from build123d import *

# Parameters (mm, degrees)
BOSS_EXTRUDE1_DEPTH = 5.08
CUT_EXTRUDE1_DEPTH  = 2.413
SKETCH8_R           = 1.524
CUT_EXTRUDE2_DEPTH  = 2.667


with BuildPart() as part:
    # Sketch1 → Boss-Extrude1 (new body)
    with BuildSketch(Plane(origin=(0, 0, 0), x_dir=(1, 0, 0), z_dir=(0, 1, 0))):
        Polygon((41.520544409, 0), (-41.520544409, 0), (-41.520544409, -3.81), (-39.615544409, -3.81), (-39.615544409, -7.112), (-44.695544409, -7.112), (-44.695544409, -3.81), (-42.790544409, -3.81), (-42.790544409, 0), (-56.515, 0), (-56.515, 107.95), (-51.435, 107.95), (-51.435, 5.08), (51.435, 5.08), (51.435, 107.95), (56.515, 107.95), (56.515, 0), (42.790544409, 0), (42.790544409, -4.019776581), (47.235544409, -4.019776581), (47.235544409, -11.639776581), (37.075544409, -11.639776581), (37.075544409, -4.019776581), (41.520544409, -4.019776581), align=None)
    extrude(amount=BOSS_EXTRUDE1_DEPTH)

    # Sketch2 → Cut-Extrude1 (cut)
    with BuildSketch(Plane(origin=(0, 5.08, 0), x_dir=(1, 0, 0), z_dir=(0, 1, 0))):
        Polygon((40.322457304, -4.654776581), (38.4893702, -7.829776581), (40.322457304, -11.004776581), (43.988631514, -11.004776581), (45.821718619, -7.829776581), (43.988631514, -4.654776581), align=None)
    extrude(amount=-CUT_EXTRUDE1_DEPTH, mode=Mode.SUBTRACT)

    # Sketch8 → Cut-Extrude2 (cut)
    with BuildSketch(Plane(origin=(0, 2.667, 0), x_dir=(1, 0, 0), z_dir=(0, 1, 0))):
        with Locations(Location((42.155544409, -7.829776581, 0), (0, 0, 270))):
            Circle(SKETCH8_R)
    extrude(amount=-CUT_EXTRUDE2_DEPTH, mode=Mode.SUBTRACT)


solid = part.part
Read the model definition and answer for the solid it produces. Units are mm, in the model's axes. A direction names the side the tool comes from. Coordinates: 2 decimals unless noted, no trailing zeros. Loops run counter-clockwise (first coordinate to the right, second up) from the corner with the lowest first, then second, coordinate; pieces in that order, holes last. Notation, with made-up numbers: (-35, 87) -> (-14, 87) arc R25 ccw to (-14, 110) -> close; hole circle Ø4 at (12, -32). An arc over 180 degrees is marked (long way). Write item = value, one per line. Start each with the question number.
1) For faces 1 (the face through (44, 2.667, 8)), 2 (the face through (41.521, 3, 2)), 3 (the face through (37.076, 3, 8)), 4 (the face through (50, 3, 0)), determine the directions among +Z, -Z, +X, -X, +Y, -Y from which every point of the face is accessible in a straight line to the end or side of a thin tool.
2) Find the intervals of material crossed by L1, parallel to X at y = 4.2, z = -13 (3 decimals); L2, parallel to Z at x = -49.5, y = 4.75; L3, parallel to X at y = 2.15, z = 1, in increasing order. Write a range as from..to.
3) Given P1, Ø1, axis at x = -43.5, y = 3, coming from the -Z side; P2, Ø1, axis at y = 3, z = 5, coming from the +X side; P3, Ø7, axis at x = 41.5, z = 7.5, coming from the +Y side; P4, Ø2.5, axis at x = -43, y = 1.5, coming from the +Z side, each flat-ended and moving along its own axis, determine where each tip first touches the part or whether it passes through.
4) The part is cut by section A-A, the plane z = -96. Determine the outline of the cut face in (x, y) (3 decimals).
5) The part is cut by section C-C, the plane x = 1. Determine the outline of the cut face in (y, z), plus the area to 3 significant figures.
6) The mould has two halves that part along X. Classify faces 5 (the face through (39, 3, 4.02)), 6 (the face through (-42, 3, 7.112)), 7 (the face through (47.236, 3, 8)), 8 (the face through (-1, 3, -5.08)): pulls with the +X half, pulls with the -X half, needs draft (parallel to the pull), parting line crosses it, or undercut.
Result:
q1.face_1 = +Y
q1.face_2 = +Y, -Y
q1.face_3 = +Z, +Y, -Y
q1.face_4 = +X, +Y, -Y
q2.L1 = -56.515..-51.435, 51.435..56.515
q2.L2 = -5.08..0
q2.L3 = -42.79..-41.52, 41.52..42.79
q3.P1 = -5.08
q3.P2 = 47.24
q3.P3 = 5.08
q3.P4 = 7.11
q4.outline = (-56.515, 0) -> (-51.435, 0) -> (-51.435, 5.08) -> (-56.515, 5.08) -> close; (51.435, 0) -> (56.515, 0) -> (56.515, 5.08) -> (51.435, 5.08) -> close
q5.outline = (0, -5.08) -> (5.08, -5.08) -> (5.08, 0) -> (0, 0) -> close
q5.area = 25.8 mm²
q6.face_5 = undercut
q6.face_6 = needs draft
q6.face_7 = pulls with the +X half
q6.face_8 = undercut
